Read the model definition and answer for the solid it produces. Units are mm, in the model's axes. Coordinates: 2 decimals unless noted, no trailing zeros. Order: outer loops, then holes, each group sorted by start corner. A loop starts at its lowest first (then second) coordinate and runs counter-clockwise, first axis right, second up. Notation, with made-up numbers: (8, 78.5) - (39, 78.5) arc R16 cw to (39, 93.5) - close; hole circle Ø6 at (31, 43.5). An arc over 180 degrees is marked (long way). Write item = value, one per line.
from build123d import *

# Parameters (mm, degrees)
SKETCH1_W           = 382.452818204
SKETCH1_H           = 50.8
SKETCH1_R           = 14.3002
SKETCH1_R_2         = 2.54
BOSS_EXTRUDE1_DEPTH = 3.175
FILLET1_R           = 7.62


with BuildPart() as part:
    # Sketch1 → Boss-Extrude1 (new body)
    with BuildSketch(Plane.XY):
        with Locations((132.2654537, 9.352736133)):
            Rectangle(SKETCH1_W, SKETCH1_H)
        with Locations((-34.334788468, 9.352736133)):
            Circle(SKETCH1_R, mode=Mode.SUBTRACT)
        with Locations((298.913211532, 9.352736133)):
            Circle(SKETCH1_R, mode=Mode.SUBTRACT)
        with Locations((53.803211532, 9.352736133)):
            Circle(SKETCH1_R, mode=Mode.SUBTRACT)
        with Locations((87.573397818, 9.352736133)):
            Circle(SKETCH1_R, mode=Mode.SUBTRACT)
        with Locations((19.729570927, 9.352736133)):
            Circle(SKETCH1_R, mode=Mode.SUBTRACT)
        with Locations((98.619809052, -9.430651268)):
            Circle(SKETCH1_R_2, mode=Mode.SUBTRACT)
        with Locations((111.319809052, -9.430651268)):
            Circle(SKETCH1_R_2, mode=Mode.SUBTRACT)
        with Locations((111.319809052, 3.269348732)):
            Circle(SKETCH1_R_2, mode=Mode.SUBTRACT)
        with Locations((111.319809052, 15.969348732)):
            Circle(SKETCH1_R_2, mode=Mode.SUBTRACT)
        with Locations((111.319809052, 28.669348732)):
            Circle(SKETCH1_R_2, mode=Mode.SUBTRACT)
        with Locations((98.619809052, 28.669348732)):
            Circle(SKETCH1_R_2, mode=Mode.SUBTRACT)
        with Locations((47.819809052, -9.430651268)):
            Circle(SKETCH1_R_2, mode=Mode.SUBTRACT)
        with Locations((60.519809052, -9.430651268)):
            Circle(SKETCH1_R_2, mode=Mode.SUBTRACT)
        with Locations((47.819809052, 28.669348732)):
            Circle(SKETCH1_R_2, mode=Mode.SUBTRACT)
        with Locations((60.519809052, 28.669348732)):
            Circle(SKETCH1_R_2, mode=Mode.SUBTRACT)
        with Locations((35.119809052, 28.669348732)):
            Circle(SKETCH1_R_2, mode=Mode.SUBTRACT)
        with Locations((9.719809052, -9.430651268)):
            Circle(SKETCH1_R_2, mode=Mode.SUBTRACT)
        with Locations((-2.980190948, -9.430651268)):
            Circle(SKETCH1_R_2, mode=Mode.SUBTRACT)
        with Locations((-2.980190948, 3.269348732)):
            Circle(SKETCH1_R_2, mode=Mode.SUBTRACT)
        with Locations((-2.980190948, 15.969348732)):
            Circle(SKETCH1_R_2, mode=Mode.SUBTRACT)
        with Locations((9.719809052, 28.669348732)):
            Circle(SKETCH1_R_2, mode=Mode.SUBTRACT)
        with Locations((-2.980190948, 28.669348732)):
            Circle(SKETCH1_R_2, mode=Mode.SUBTRACT)
        with Locations((156.877176863, 9.352736133)):
            Circle(SKETCH1_R_2, mode=Mode.SUBTRACT)
        with Locations((169.577176863, 9.352736133)):
            Circle(SKETCH1_R_2, mode=Mode.SUBTRACT)
        with Locations((182.277176863, 9.352736133)):
            Circle(SKETCH1_R_2, mode=Mode.SUBTRACT)
        with Locations((194.977176863, 9.352736133)):
            Circle(SKETCH1_R_2, mode=Mode.SUBTRACT)
        with Locations((207.677176863, 9.352736133)):
            Circle(SKETCH1_R_2, mode=Mode.SUBTRACT)
    extrude(amount=BOSS_EXTRUDE1_DEPTH)

    # Fillet1
    fillet1_edges = [part.edges().sort_by_distance(p)[0] for p in [
        (-58.960955402, 34.752736133, 1.5875),
        (323.491862802, 34.752736133, 1.5875),
        (323.491862802, -16.047263867, 1.5875),
        (-58.960955402, -16.047263867, 1.5875),
    ]]
    fillet(fillet1_edges, radius=FILLET1_R)


solid = part.part
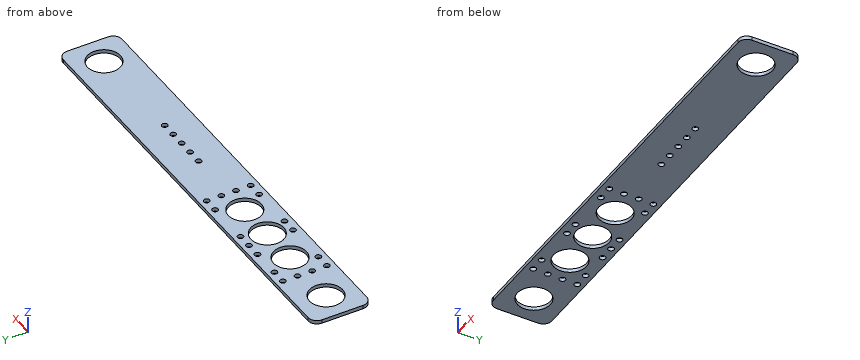
1) The part is cut by section B-B (z = 1.2). Count the separate pieces of the cut face and the enclosed holes in it, and give its area (3 significant figures).
Returned:
separate_pieces = 1
enclosed_holes = 27
area = 15,700 mm^2
2) Straight lines are drawn through the part: line 1 along Y through (x, z) = (156.5, 1.3); line 2 along X through (y, z) = (12.5, 2.25); line 3 along Y through (x, z) = (9.5, 1.25). For each, find the intervals that lie inside material, in ascending order. Write a range as from..to.
Returned:
line_1 = -16.05..6.84, 11.86..34.75
line_2 = -58.96..-48.28, -20.39..5.78, 33.68..39.85, 67.75..73.62, 101.52..284.96, 312.86..323.49
line_3 = -16.05..-11.96, -6.9..-0.64, 19.35..26.14, 31.2..34.75
3) Flat-ended cylindrical pins translate along their axes: pin 1 Ø12 at (x, y) = (14, 13) entering from -Z; pin 2 Ø1.5 at (y, z) = (28.5, 0.5) entering from +X. Find the tip coordinate at first contact, or state that the pin passes through.
Returned:
pin_1 = through
pin_2 = 323.47
4) The part is cut by section A-A (x = 289.5). Determine the outline of the cut face in (y, z) (3 decimals), and give its area (3 significant figures).
Returned:
outline = (-16.047, 0) - (-1.412, 0) - (-1.412, 3.175) - (-16.047, 3.175) - close; (20.118, 0) - (34.753, 0) - (34.753, 3.175) - (20.118, 3.175) - close
area = 92.9 mm^2
